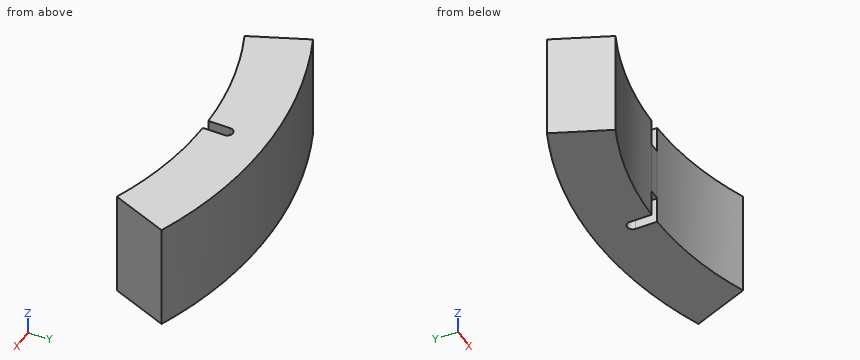
from build123d import *

# Parameters (mm, degrees)
BOSS_EXTRUDE3_DEPTH      = 20
BOSS_EXTRUDE3_DEPTH_BACK = 20
SKETCH2_8_R              = 1.25
BOSS_EXTRUDE5_DEPTH      = 10
BOSS_EXTRUDE5_DEPTH_BACK = 10


with BuildPart() as part:
    # Sketch2 → Boss-Extrude3 (new body, two sides)
    with BuildSketch(Plane.XY.offset(11)) as boss_extrude3_sk:
        with BuildLine():
            ThreePointArc((2, 119.983332176), (24.390845035, 117.495049591), (45.922011884, 110.865543901))
            Line((45.922011884, 110.865543901), (54.532389112, 131.652833383))
            ThreePointArc((54.532389112, 131.652833383), (0, 142.5), (-54.532389112, 131.652833383))
            Line((-54.532389112, 131.652833383), (-45.922011884, 110.865543901))
            ThreePointArc((-45.922011884, 110.865543901), (-24.390845035, 117.495049591), (-2, 119.983332176))
            Line((-2, 119.983332176), (-2, 128))
            ThreePointArc((-2, 128), (0, 130), (2, 128))
            Line((2, 128), (2, 119.983332176))
        make_face()
    extrude(amount=BOSS_EXTRUDE3_DEPTH)
    extrude(boss_extrude3_sk.sketch, amount=-BOSS_EXTRUDE3_DEPTH_BACK)

    # Sketch2_8 → Boss-Extrude5 (add, two sides)
    with BuildSketch(Plane.XY.offset(11)) as boss_extrude5_sk:
        with BuildLine():
            ThreePointArc((-2, 119.983332176), (0, 120), (2, 119.983332176))
            Line((2, 119.983332176), (2, 128))
            ThreePointArc((2, 128), (0, 130), (-2, 128))
            Line((-2, 128), (-2, 119.983332176))
        make_face()
        with Locations((0, 128)):
            Circle(SKETCH2_8_R, mode=Mode.SUBTRACT)
    extrude(amount=BOSS_EXTRUDE5_DEPTH)
    extrude(boss_extrude5_sk.sketch, amount=-BOSS_EXTRUDE5_DEPTH_BACK)


solid = part.part
Design review of the part built by this model. Coordinates are the model's own, in mm. Round coordinates to 2 decimals unless told otherwise and drop trailing zeros. Write each loop counter-clockwise with the first axis right and the second up, starting at its lowest first coordinate (ties: lowest second). Pieces come first, ordered by that corner, then holes. Notation, with made-up numbers: M -18,-17.75 L 21,-17.75 A29 ccw 21,9.25 Z; hole C -29,2 d6. An arc over 180 degrees is marked long. One line per item, written item: value. Start each with the question number.
1. To check wall thickness, follow probe 1 along Y at (x, z) = (0, 15); probe 2 along X at (y, z) = (128, 16); probe 3 along Y at (x, z) = (41.5, -3). State the ranges of each line that lie inside material, in increasing order. Write a range as from..to.
2. Take a section at D-D on z = -3. State the section outline as (x, y) points, then the cut area to 3 significant figures.
3. Clearance check with flat-ended pins moving along their axes: P1, Ø10, axis at x = -39.5, z = -1.5, coming from the -Y side; P2, Ø8, axis at x = -35, z = 6, coming from the -Y side; P3, Ø1.5, axis at y = 131, z = 3.5, coming from the +X side; P4, Ø4, axis at y = 128.5, z = 25, coming from the +X side. State where each tip first meets the part, or that it passes through.
4. Take a section at B-B on x = 0. State the section outline as (y, z) points, then the cut area to 3 significant figures.
5. Take a section at C-C on y = 118.5. State the section outline as (x, z) points.
6. Take a section at A-A on z = 20. State the section outline as (x, y) points, then the cut area to 3 significant figures.
Computed:
1. probe 1: y = 120..126.75, 129.25..142.5
1. probe 2: x = -53.02..-1.25, 1.25..53.02
1. probe 3: y = 112.6..136.32
2. outline: M -54.53,131.65 L -45.92,110.87 A120 cw -2,119.98 L -2,128 A2 cw 2,128 L 2,119.98 A120 cw 45.92,110.87 L 54.53,131.65 A142.5 ccw Z
2. area: 2,280 mm²
3. P1: stops at y = 111.44
3. P2: stops at y = 113.49
3. P3: stops at x = 54.53
3. P4: stops at x = 54.05
4. outline: M 120,1 L 126.75,1 L 126.75,21 L 120,21 Z; M 129.25,1 L 130,1 L 130,-9 L 142.5,-9 L 142.5,31 L 130,31 L 130,21 L 129.25,21 Z
4. area: 650 mm²
5. outline: M -49.08,-9 L -18.91,-9 L -18.91,31 L -49.08,31 Z; M 18.91,-9 L 49.08,-9 L 49.08,31 L 18.91,31 Z
6. outline: M -54.53,131.65 L -45.92,110.87 A120 cw -2,119.98 A120 cw 2,119.98 A120 cw 45.92,110.87 L 54.53,131.65 A142.5 ccw Z; hole C 0,128 d2.5
6. area: 2,310 mm²
